For this review, take the finished solid that the model builds, in its own axes (mm). A direction names the side the tool comes from. Coordinates: 2 decimals unless noted, no trailing zeros. Write each loop counter-clockwise with the first axis right and the second up, starting at its lowest first coordinate (ties: lowest second). Pieces come first, ordered by that corner, then holes.
1) Mouldability with a two-part tool opening along X and no side actions: class faces 1 (the face through (14, 0, 17)), 2 (the face through (-11.25, 0, 20)), 3 (the face through (5, 0, 29.5)) as pulls with the +X half, pulls with the -X half, needs draft (parallel to the pull), parting line crosses it, or undercut.
2) We need section B-B on x = 13.5. Write out the cut boundary in (y, z).
3) We need section D-D on x = 4.75. Write out the cut boundary in (y, z), then the cut area to 3 significant figures.
4) Insertion check: P1, Ø0.9, axis at x = 22.5, z = 7.5, coming from the +Y side; P2, Ø4, axis at x = 14, y = -2, coming from the +Z side; P3, Ø1.5, axis at x = 18.5, z = 8, coming from the -Y side. Each pin has a flat end and moves straight along its axis. Give the tip position at first contact, or say it passes through.
5) We need section C-C on z = 13.25. Write out the cut boundary in (x, y).
6) We need section A-A on x = -13.5. Write out the cut boundary in (y, z), then the cut area to 3 significant figures.
7) For faces 4 (the face through (-15, 0, 18.5)), 5 (the face through (21, 0, 6)), 6 (the face through (5.9, -2.4, 26.5)), list the 3-axis set-ups (+Z, -Z, +X, -X, +Y, -Y) from which the entire face can be reached by the end or side of a thin tool; tool diameter is ignored.
8) To check wall thickness, follow line 1 along X through (y, z) = (0, 17.1); line 2 along Y through (x, z) = (13.5, 17.35); line 3 along Z through (x, y) = (15.5, 1). State the ranges of each line that lie inside material, in increasing order.
Autodesk Inventor part; units mm, degrees
ref_plane "YZ Plane" through (0, 0, 0) normal (1, 0, 0) x (0, 1, 0)
ref_plane "XZ Plane" through (0, 0, 0) normal (0, 1, 0) x (-1, 0, 0)
ref_plane "XY Plane" through (0, 0, 0) normal (0, 0, 1) x (1, 0, 0)
sketch "Skizze1" plane through (0, 0, 0) normal (0, 1, 0) x (-1, 0, 0)
  line L0 (-11.25, 0) -> (11.25, 0)
  line L1 (11.25, 0) -> (11.25, 16)
  line L2 (11.25, 16) -> (16.25, 16)
  line L3 (16.25, 16) -> (16.25, 18.5)
  line L4 (16.25, 18.5) -> (11.25, 18.5)
  line L5 (11.25, 18.5) -> (11.25, 22.5)
  line L6 (11.25, 22.5) -> (0, 22.5)
  line L7 (0, -4.5) -> (0, 27)
  line L8 (-11.25, 0) -> (-11.25, 16)
  line L9 (-11.25, 16) -> (-16.25, 16)
  line L10 (-16.25, 16) -> (-16.25, 18.5)
  line L11 (-16.25, 18.5) -> (-11.25, 18.5)
  line L12 (-11.25, 18.5) -> (-11.25, 22.5)
  line L13 (-11.25, 22.5) -> (0, 22.5)
  point P0 (0, 0)
  dimension "d0" = 22.5
  dimension "d1" = 16
  dimension "d2" = 5
  dimension "d3" = 2.5
  dimension "d4" = 4
  dimension "d5" = 0
extrude "Extrusion1" add sketch "Skizze1" along normal mid plane 12
fillet "Rundung1" radius 0.5 29 edges at (0, -6, 22.5) (11.25, 0, 0) (11.25, -6, 8) (11.25, -6, 20.5) (11.25, 6, 20.5) (-11.25, 0, 22.5) (11.25, 0, 22.5) (0, 6, 22.5) (-11.25, -6, 8) (-11.25, -6, 20.5) (-13.75, -6, 18.5) (-13.75, -6, 16) (-16.25, -6, 17.25) (13.75, -6, 18.5) (13.75, -6, 16) (16.25, 0, 16) (16.25, 0, 18.5) (16.25, 6, 17.25) (11.25, 6, 8) (-11.25, 6, 20.5) (-13.75, 6, 18.5) (-16.25, 6, 17.25) (-16.25, 0, 18.5) (-16.25, 0, 16) (-13.75, 6, 16) (-11.25, 6, 8) (-11.25, 0, 0) (0, 6, 0) (0, -6, 0)
sketch "Skizze2" plane through (-10.75, 5.5, 22.5) normal (0, 0, 1) x (1, 0, 0)
  circle A0 centre (15.5, -5.5) radius 6
  line L0 (21.5, 0) -> (21.5, -11)
  line L1 (21.5, 0.5) -> (0, 0.5)
  point P0 (10.75, -5.5)
  point P1 (21.5, -5.5)
  point P2 (21.5, -5.5)
  dimension "d9" = 6
extrude "Extrusion2" add sketch "Skizze2" along normal blind 4
sketch "Skizze3" plane through (4.75, 0, 26.5) normal (0, 0, 1) x (1, 0, 0)
  circle A0 centre (0, 0) radius 2.5
  arc A1 (2.3979, 5.5) -> (-2.3979, 5.5) centre (0, 0) ccw
  point P0 (0, 6)
  point P1 (6, 0)
  dimension "d14" = 5
extrude "Extrusion3" add sketch "Skizze3" along normal blind 3
fillet "Rundung2" radius 0.5 1 edges at (-1.25, 0, 26.5)
chamfer "Fasen1" distance 0.3 angle 45 1 edges at (2.25, 0, 29.5)
sketch "Skizze4" plane through (11.25, -5.5, 0.5) normal (1, 0, 0) x (0, 0, -1)
  line L0 (-8.5, 1.5) -> (-5.5, 1.5)
  line L1 (-5.5, 1.5) -> (-5.5, 9.5)
  line L2 (-5.5, 9.5) -> (-8.5, 9.5)
  line L3 (-8.5, 9.5) -> (-8.5, 1.5)
  line L4 (0.5, 0) -> (0.5, 11)
  point P0 (0.5, 5.5)
  point P1 (-5.5, 5.5)
  point P2 (0.5, 5.5)
  dimension "d21" = 8
  dimension "d22" = 3
  dimension "d23" = 6
extrude "Extrusion4" add sketch "Skizze4" along normal blind 20
sketch "Skizze5" plane through (10.75, 6, 18.5) normal (0, 0, 1) x (1, 0, 0)
  circle A0 centre (-6, -6) radius 2.2
  line L0 (-26.5, -0.5) -> (-22, -0.5)
  point P0 (-10.75, -6)
  point P1 (2.75, -6)
  point P2 (-24.25, -6)
  point P3 (-24.25, -0.5)
  dimension "d26" = 27
hole "Bohrung1" at (13.5, 0, 18.5) at (-13.5, 0, 18.5) direction (0, 0, -1) diameter 1 depth 8 tip angle 118
properties part number "Motor"
Result:
1. face 1: undercut
1. face 2: pulls with the -X half
1. face 3: needs draft
2. outline: (-6, 16.5) arc R0.5 ccw to (-5.5, 16) - (-0.5, 16) - (-0.5, 18.5) - (-5.5, 18.5) arc R0.5 ccw to (-6, 18) - close; (-4, 6) - (4, 6) - (4, 9) - (-4, 9) - close; (0.5, 16) - (6, 16) - (6, 18.5) - (0.5, 18.5) - close
3. outline: (-6, 0.5) arc R0.5 ccw to (-5.5, 0) - (5.5, 0) arc R0.5 ccw to (6, 0.5) - (6, 22) arc R0.5 ccw to (5.5, 22.5) - (6, 22.5) - (6, 26) arc R0.5 ccw to (5.5, 26.5) - (2.5, 26.5) - (2.5, 29.2) - (2.2, 29.5) - (-2.2, 29.5) - (-2.5, 29.2) - (-2.5, 26.5) - (-5.5, 26.5) arc R0.5 ccw to (-6, 26) - (-6, 22.5) - (-5.5, 22.5) arc R0.5 ccw to (-6, 22) - close
3. area: 333 mm2
4. P1: stops at y = 4
4. P2: stops at z = 18.5
4. P3: stops at y = -4
5. outline: (-11.25, -5.5) arc R0.5 ccw to (-10.75, -6) - (10.75, -6) arc R0.5 ccw to (11.25, -5.5) - (11.25, 5.5) arc R0.5 ccw to (10.75, 6) - (-10.75, 6) arc R0.5 ccw to (-11.25, 5.5) - close
6. outline: (-6, 16.5) arc R0.5 ccw to (-5.5, 16) - (-0.5, 16) - (-0.5, 18.5) - (-5.5, 18.5) arc R0.5 ccw to (-6, 18) - close; (0.5, 16) - (5.5, 16) arc R0.5 ccw to (6, 16.5) - (6, 18) arc R0.5 ccw to (5.5, 18.5) - (0.5, 18.5) - close
6. area: 27.3 mm2
7. face 4: +Z, -X, +Y, -Y
7. face 5: -Z, +X, +Y, -Y
7. face 6: +Z
8. line 1: x = -16.25 to -14, -13 to 13, 14 to 16.25
8. line 2: y = -6 to -0.5, 0.5 to 6
8. line 3: z = 6 to 9, 16 to 18.5
